Autodesk Inventor part; units mm, degrees
ref_plane "YZ Plane" through (0, 0, 0) normal (1, 0, 0) x (0, 1, 0)
ref_plane "XZ Plane" through (0, 0, 0) normal (0, 1, 0) x (-1, 0, 0)
ref_plane "XY Plane" through (0, 0, 0) normal (0, 0, 1) x (1, 0, 0)
sketch "Sketch1" plane through (0, 0, 0) normal (0, 0, 1) x (1, 0, 0)
  line L0 (0, 0) -> (4, 0)
  line L1 (4, 0) -> (4, 4)
  line L2 (4, 4) -> (0, 4)
  line L3 (0, 4) -> (0, 0)
  dimension "d0" = 4
  dimension "d1" = 4
extrude "Extrusion1" add sketch "Sketch1" along normal blind 128.5
sketch "Sketch3" plane through (0, 0, 128.5) normal (0, 0, 1) x (1, 0, 0)
  line L0 (0, 0) -> (4, 0)
  line L1 (-3.5, 0) -> (7.5, 0)
  line L2 (7.5, 0) -> (7.5, 8)
  line L3 (7.5, 8) -> (-3.5, 8)
  line L4 (-3.5, 8) -> (-3.5, 0)
  point P0 (2, 0)
  dimension "d4" = 11
  dimension "d5" = 8
extrude "Extrusion2" add sketch "Sketch3" along normal blind 11.5
sketch "Sketch4" plane through (0, 0, 0) normal (0, -1, 0) x (1, 0, 0)
  line L0 (7.5, 128.5) -> (7.5, 140)
  line L1 (-3.5, 140) -> (7.5, 140)
  line L2 (-1.75, 136) -> (5.75, 136)
  line L3 (5.75, 136) -> (5.75, 132.5)
  line L4 (5.75, 132.5) -> (-1.75, 132.5)
  line L5 (-1.75, 132.5) -> (-1.75, 136)
  point P0 (2, 136)
  point P1 (2, 140)
  point P2 (5.75, 134.25)
  point P3 (7.5, 134.25)
  dimension "d8" = 7.5
  dimension "d9" = 3.5
extrude "Extrusion3" cut sketch "Sketch4" against normal blind 8
sketch "Sketch5" plane through (0, 0, 140) normal (0, 0, 1) x (1, 0, 0)
  circle A0 centre (2, 4) radius 2.1
  point P0 (0, 0)
  dimension "d12" = 4.2
extrude "Extrusion4" cut sketch "Sketch5" against normal up to surface (7.5 mm away)
sketch "Sketch6" plane through (-3.5, 8, 128.5) normal (0, 1, 0) x (1, 0, 0)
  line L0 (11, 0) -> (0, 0)
  line L1 (0, 0) -> (0, -11.5)
  line L2 (11, -11.5) -> (0, -11.5)
  line L3 (11, 0) -> (11, -11.5)
  point P0 (3.5, 128.5)
extrude "Extrusion5" add sketch "Sketch6" along normal blind 1
mirror "Mirror2" about plane through (0, 0, 0) normal (0, 0, 1) of "Extrusion1", "Extrusion5", "Extrusion2", "Extrusion3", "Extrusion4"
sketch "Sketch7" plane through (0, 0, 140) normal (0, 0, 1) x (1, 0, 0)
  line L0 (-3.5, 0) -> (7.5, 0)
  arc A0 (4.0616, 0) -> (-0.0616, 0) centre (2, 4) ccw
  line L1 (0, 0) -> (-0.0616, 0)
  line L2 (-0.0616, 0) -> (4.0616, 0)
  circle A1 centre (2, 4) radius 3.25
  dimension "d17" = 9
  dimension "d18" = 6.5
extrude "Extrusion6" add sketch "Sketch7" along normal blind 2.5
sketch "Sketch8" plane through (-3.5, 8, 128.5) normal (0, -1, 0) x (1, 0, 0)
  line L0 (1.75, 7.5) -> (1.75, 4)
  line L1 (1.75, 4) -> (9.25, 4)
  line L2 (9.25, 4) -> (9.25, 7.5)
  line L3 (9.25, 7.5) -> (1.75, 7.5)
  point P0 (3.5, -128.5)
mirror "Mirror3" about plane through (0, 0, 0) normal (0, 0, 1) of "Extrusion6"
sketch "Sketch10" plane through (-3.5, 9, -128.5) normal (0, 1, 0) x (1, 0, 0)
  line L0 (0, 0) -> (11, 0)
  line L1 (11, 0) -> (11, -9)
  line L2 (11, -9) -> (0, -9)
  line L3 (0, -9) -> (0, 0)
  point P0 (3.5, -128.5)
  dimension "d21" = 9
extrude "Extrusion7" add sketch "Sketch10" against normal up to surface (9 mm away)
sketch "Sketch11" plane through (-3.5, 9, -140) normal (0, 1, 0) x (1, 0, 0)
  line L0 (11, -20.5) -> (0, -20.5)
  circle A0 centre (5.5, -15) radius 2.1
  point P0 (3.5, -140)
  dimension "d24" = 4.2
  dimension "d25" = 5.5
extrude "Extrusion8" cut sketch "Sketch11" against normal blind 11
sketch "Sketch12" plane through (-3.5, 0, -140) normal (-1, 0, 0) x (0, 0, 1)
  line L0 (20.5, 9) -> (20.5, 0)
  line L1 (18.75, 6.25) -> (11.25, 6.25)
  line L2 (11.25, 6.25) -> (11.25, 2.75)
  line L3 (11.25, 2.75) -> (18.75, 2.75)
  line L4 (18.75, 2.75) -> (18.75, 6.25)
  point P0 (140, 0)
  point P1 (18.75, 4.5)
  point P2 (20.5, 4.5)
  dimension "d28" = 7.5
  dimension "d29" = 3.5
  dimension "d30" = 1.75
extrude "Extrusion9" cut sketch "Sketch12" against normal blind 11
fillet "Fillet3" radius 0.5 1 edges at (2, 8.5, -140)
sketch "Sketch14" plane through (-3.5, 9, -119.5) normal (0, 0, 1) x (1, 0, 0)
  line L0 (7.5, -9) -> (7.5, -5)
  line L1 (7.5, -9) -> (11, -9)
  line L2 (11, 0) -> (11, -9)
  line L3 (11, 0) -> (0, 0)
  line L4 (0, 0) -> (0, -9)
  line L5 (0, -9) -> (3.5, -9)
  line L6 (3.5, -5) -> (3.5, -9)
  line L7 (7.5, -5) -> (3.5, -5)
extrude "Extrusion10" add sketch "Sketch14" along normal blind 2
fillet "Fillet4" radius 1.5 3 edges at (4, 2, -117.5) (2, 4, -117.5) (0, 2, -117.5)
mirror "Mirror5" about plane through (0, 0, 0) normal (0, 0, 1) of "Extrusion7", "Extrusion8", "Extrusion9", "Extrusion10"
fillet "Fillet5" radius 1.5 3 edges at (0, 2, 117.5) (2, 4, 117.5) (4, 2, 117.5)
fillet "Fillet6" radius 0.5 1 edges at (2, 8.5, 140)
properties part number "Axle280mm"
Geometry check sheet. Reference: the model listing, model coordinates, mm. A direction names the side the tool comes from. Give positions to 0.01 mm unless a question says otherwise; leave off trailing zeros. Order: outer loops, then holes, each group sorted by start corner. A loop starts at its lowest first (then second) coordinate and runs counter-clockwise, first axis right, second up. Notation, with made-up numbers: (35.25, 11) - (41.25, 11) arc R20 cw to (41.25, 19) - close; hole circle Ø3 at (67, 79.25). An arc over 180 degrees is marked (long way). Write item = value, one per line. Start each with the question number.
1) Scan lines: L1, parallel to Z at x = 2, y = 1.1; L2, parallel to Z at x = 6, y = 3; L3, parallel to Z at x = 2, y = 6.9. Record each from-to range of solid material in increasing order.
2) Section check A-A (z = 21). Enter the section's corners in (x, y).
3) Access from +Z, -Z, +X, -X, +Y, -Y to the whole of each face (thin tool, end or side, straight path). Record for faces 4 (the cylindrical face through (2.168, 8.497, -141.486)), 5 (the flat face through (-3, 5.5, 140)), 6 (the flat face through (-1, 2.75, -125)), 7 (the flat face through (-3.2, 5.1, -140)), 8 (the flat face through (0, 6, 136)).
4) Draft check along Z on faces 1 (the flat face through (-1, 2.75, 125)), 2 (the flat face through (2.77, 6.12, 140)), 3 (the flat face through (2, 9, -129)). Enter one of: released by +Z, released by -Z, zero draft, split by the parting line, or undercut.
5) Gauge pin test, flat ends, axial feed: pin 1 Ø4.5 at (x, y) = (2.5, 3.5) entering from +Z; pin 2 Ø1.2 at (y, z) = (2, -32.5) entering from -X; pin 3 Ø4.5 at (y, z) = (1, 52) entering from +X. Record the tip position at first contact, or that the pin passes through.
Geometry check:
q1.L1 = -140 to -136, -132.5 to -127.1, -122.9 to 122.9, 127.1 to 132.5, 136 to 140
q1.L2 = -142.5 to -128.75, -121.25 to -117.5, 117.5 to 121.25, 128.75 to 142.5
q1.L3 = -140 to -136, -132.5 to -127.1, -122.9 to -117.5, 117.5 to 122.9, 127.1 to 132.5, 136 to 140
q2.outline = (0, 0) - (4, 0) - (4, 4) - (0, 4) - close
q3.face_4 = -Z
q3.face_5 = +Z, -X
q3.face_6 = +X, -X
q3.face_7 = -Z, -X
q3.face_8 = -Y
q4.face_1 = undercut
q4.face_2 = released by +Z
q4.face_3 = zero draft
q5.pin_1 = 140
q5.pin_2 = 0
q5.pin_3 = 4
